Source: CAD feature listing. Evaluate the final solid. Frame: model axes, mm. A direction names the side the tool comes from. Give positions to 0.01 mm unless a question says otherwise; leave off trailing zeros. Write each loop counter-clockwise with the first axis right and the second up, starting at its lowest first coordinate (ties: lowest second). Pieces come first, ordered by that corner, then holes. Notation, with made-up numbers: (-36.75, 13) -> (22.25, 13) arc R15 cw to (22.25, 17) -> close; hole circle Ø10 at (-8, 9.25). An arc over 180 degrees is marked (long way). Answer as a JSON object with one key per item and string values. Group by question number.
Item 1: First-contact query: pin 1 Ø1.5 at (x, y) = (-183.5, 3.5) entering from -Z; pin 2 Ø1.5 at (x, y) = (132, 2) entering from +Z; pin 3 Ø3 at (x, z) = (-211.5, -104.5) entering from -Y. Flat tips, straight axial feed; report the tip coordinate or a pass-through.
Item 2: Section query A-A on x = 87.5. Return the cut outline in (y, z).
Item 3: Section query C-C on y = 4.1. Give the number of separate pieces and of enclosed holes in the cut face, plus the area to 3 significant figures.
Item 4: Ray query, probe 1 along Z at (x, y) = (-6, 3.85); probe 2 along X at (y, z) = (4.05, 16); probe 3 along X at (y, z) = (4.35, 125). Return the intervals inside material, ascending. Write a range as from..to.
Item 5: Pull-direction query (Z, two-part tool) for faces 3 (the face through (-193.081, 2.465, 118.033)), 4 (the face through (-174.6, 2.46, -43.16)), 5 (the face through (-41, 0, 72)), 6 (the face through (241.15, 2.46, -140.99)); classes: pulls with the +Z half, pulls with the -Z half, needs draft (parallel to the pull), parting line crosses it, or undercut.
Item 6: Access query for faces 1 (the face through (-41, 5, 72)), 2 (the face through (-217.63, 2.46, 81.57)). Directions: +Z, -Z, +X, -X, +Y, -Y. A direction counts if a zero-diameter tool reaches every point of the face in a straight line with its end or side. Return the directions, or none.
Item 7: Section query B-B on z = 16. Return the cut outline in (x, y), plus the area to 3 significant figures.
from build123d import *

# Parameters (mm, degrees)
ESQUISSE1_R        = 1.75
ESQUISSE1_R_2      = 11.5
ESQUISSE1_R_3      = 2.25
BOSS_EXTRU_1_DEPTH = 5


with BuildPart() as part:
    # Esquisse1 → Boss.-Extru.1 (new body)
    with BuildSketch(Plane(origin=(0, 0, 0), x_dir=(1, 0, 0), z_dir=(0, 1, 0))):
        with BuildLine():
            Line((-196.5, -144), (196.5, -144))
            ThreePointArc((196.5, -144), (201.644957554, -145.425070743), (205.323529412, -149.294117647))
            ThreePointArc((205.323529412, -149.294117647), (256.980970389, -156.980970389), (249.294117647, -105.323529412))
            ThreePointArc((249.294117647, -105.323529412), (245.425070743, -101.644957554), (244, -96.5))
            Line((244, -96.5), (244, 134))
            ThreePointArc((244, 134), (241.071067812, 141.071067812), (234, 144))
            Line((234, 144), (39.764934301, 144))
            ThreePointArc((39.764934301, 144), (34.076969712, 145.775216792), (30.408479172, 150.470588235))
            ThreePointArc((30.408479172, 150.470588235), (0, 171.5), (-30.408479172, 150.470588235))
            ThreePointArc((-30.408479172, 150.470588235), (-34.076969712, 145.775216792), (-39.764934301, 144))
            Line((-39.764934301, 144), (-234, 144))
            ThreePointArc((-234, 144), (-241.071067812, 141.071067812), (-244, 134))
            Line((-244, 134), (-244, -96.5))
            ThreePointArc((-244, -96.5), (-245.425070743, -101.644957554), (-249.294117647, -105.323529412))
            ThreePointArc((-249.294117647, -105.323529412), (-256.980970389, -156.980970389), (-205.323529412, -149.294117647))
            ThreePointArc((-205.323529412, -149.294117647), (-201.644957554, -145.425070743), (-196.5, -144))
        make_face()
        with Locations(Location((-2.5, 104.5, 0), (0, 0, 270))):  # turned: the seam where the file's is
            Circle(ESQUISSE1_R, mode=Mode.SUBTRACT)
        with Locations(Location((-211.5, 104.5, 0), (0, 0, 270))):  # turned: the seam where the file's is
            Circle(ESQUISSE1_R, mode=Mode.SUBTRACT)
        with Locations(Location((211.5, 104.5, 0), (0, 0, 90))):  # turned: the seam where the file's is
            Circle(ESQUISSE1_R, mode=Mode.SUBTRACT)
        with Locations(Location((2.5, 104.5, 0), (0, 0, 270))):  # turned: the seam where the file's is
            Circle(ESQUISSE1_R, mode=Mode.SUBTRACT)
        with Locations(Location((2.5, -104.5, 0), (0, 0, 90))):  # turned: the seam where the file's is
            Circle(ESQUISSE1_R, mode=Mode.SUBTRACT)
        with Locations(Location((-2.5, -104.5, 0), (0, 0, 90))):  # turned: the seam where the file's is
            Circle(ESQUISSE1_R, mode=Mode.SUBTRACT)
        with Locations(Location((-211.5, -104.5, 0), (0, 0, 90))):  # turned: the seam where the file's is
            Circle(ESQUISSE1_R, mode=Mode.SUBTRACT)
        with Locations(Location((211.5, -104.5, 0), (0, 0, 270))):  # turned: the seam where the file's is
            Circle(ESQUISSE1_R, mode=Mode.SUBTRACT)
        with Locations(Location((0, 139, 0), (0, 0, 270))):  # turned: the seam where the file's is
            Circle(ESQUISSE1_R_2, mode=Mode.SUBTRACT)
        with Locations(Location((-234, -134, 0), (0, 0, 270))):  # turned: the seam where the file's is
            Circle(ESQUISSE1_R_2, mode=Mode.SUBTRACT)
        with Locations(Location((234, -134, 0), (0, 0, 270))):  # turned: the seam where the file's is
            Circle(ESQUISSE1_R_2, mode=Mode.SUBTRACT)
        with Locations(Location((-11.787470042, 127.212529958, 0), (0, 0, 270))):  # turned: the seam where the file's is
            Circle(ESQUISSE1_R_3, mode=Mode.SUBTRACT)
        with Locations(Location((-11.787470042, 150.787470042, 0), (0, 0, 270))):  # turned: the seam where the file's is
            Circle(ESQUISSE1_R_3, mode=Mode.SUBTRACT)
        with Locations(Location((11.787470042, 150.787470042, 0), (0, 0, 270))):  # turned: the seam where the file's is
            Circle(ESQUISSE1_R_3, mode=Mode.SUBTRACT)
        with Locations(Location((11.787470042, 127.212529958, 0), (0, 0, 270))):  # turned: the seam where the file's is
            Circle(ESQUISSE1_R_3, mode=Mode.SUBTRACT)
        with Locations(Location((-234, -117.33, 0), (0, 0, 270))):  # turned: the seam where the file's is
            Circle(ESQUISSE1_R_3, mode=Mode.SUBTRACT)
        with Locations(Location((-217.33, -134, 0), (0, 0, 270))):  # turned: the seam where the file's is
            Circle(ESQUISSE1_R_3, mode=Mode.SUBTRACT)
        with Locations(Location((-234, -150.67, 0), (0, 0, 270))):  # turned: the seam where the file's is
            Circle(ESQUISSE1_R_3, mode=Mode.SUBTRACT)
        with Locations(Location((-250.67, -134, 0), (0, 0, 270))):  # turned: the seam where the file's is
            Circle(ESQUISSE1_R_3, mode=Mode.SUBTRACT)
        with Locations(Location((234, -117.33, 0), (0, 0, 270))):  # turned: the seam where the file's is
            Circle(ESQUISSE1_R_3, mode=Mode.SUBTRACT)
        with Locations(Location((250.67, -134, 0), (0, 0, 270))):  # turned: the seam where the file's is
            Circle(ESQUISSE1_R_3, mode=Mode.SUBTRACT)
        with Locations(Location((234, -150.67, 0), (0, 0, 270))):  # turned: the seam where the file's is
            Circle(ESQUISSE1_R_3, mode=Mode.SUBTRACT)
        with Locations(Location((217.33, -134, 0), (0, 0, 270))):  # turned: the seam where the file's is
            Circle(ESQUISSE1_R_3, mode=Mode.SUBTRACT)
        with BuildLine():
            Line((-190.881530392, 107.422917163), (-125.788799552, 32.872268168))
            ThreePointArc((-125.788799552, 32.872268168), (-118.210341928, 29.449455568), (-110.663506177, 32.94143727))
            Line((-110.663506177, 32.94143727), (-46.762949895, 107.492086265))
            ThreePointArc((-46.762949895, 107.492086265), (-45.270386934, 118.178568095), (-54.355515919, 124))
            Line((-54.355515919, 124), (-183.34880304, 124))
            ThreePointArc((-183.34880304, 124), (-192.452945734, 118.13697786), (-190.881530392, 107.422917163))
        make_face(mode=Mode.SUBTRACT)
        with BuildLine():
            Line((54.355515919, 124), (183.34880304, 124))
            ThreePointArc((183.34880304, 124), (192.452945734, 118.13697786), (190.881530392, 107.422917163))
            Line((190.881530392, 107.422917163), (125.788799552, 32.872268168))
            ThreePointArc((125.788799552, 32.872268168), (118.210341928, 29.449455568), (110.663506177, 32.94143727))
            Line((110.663506177, 32.94143727), (46.762949895, 107.492086265))
            ThreePointArc((46.762949895, 107.492086265), (45.270386934, 118.178568095), (54.355515919, 124))
        make_face(mode=Mode.SUBTRACT)
        with BuildLine():
            Line((-183.930198367, -124), (-50.65119696, -124))
            ThreePointArc((-50.65119696, -124), (-41.547054266, -118.13697786), (-43.118469608, -107.422917163))
            Line((-43.118469608, -107.422917163), (-110.373862185, -30.395373528))
            ThreePointArc((-110.373862185, -30.395373528), (-117.95231981, -26.972560928), (-125.49915556, -30.46454263))
            Line((-125.49915556, -30.46454263), (-191.52276439, -107.492086265))
            ThreePointArc((-191.52276439, -107.492086265), (-193.015327352, -118.178568095), (-183.930198367, -124))
        make_face(mode=Mode.SUBTRACT)
        with BuildLine():
            Line((-206.407433976, -78.759811829), (-143.545283572, -5.420636357))
            ThreePointArc((-143.545283572, -5.420636357), (-141.137954159, 1.13300765), (-143.605122244, 7.664360214))
            Line((-143.605122244, 7.664360214), (-206.467272648, 79.660327344))
            ThreePointArc((-206.467272648, 79.660327344), (-217.512315937, 82.446130641), (-224, 73.083244507))
            Line((-224, 73.083244507), (-224, -72.251898095))
            ThreePointArc((-224, -72.251898095), (-217.469462477, -81.630748244), (-206.407433976, -78.759811829))
        make_face(mode=Mode.SUBTRACT)
        with BuildLine():
            Line((16.237050105, 97.007913735), (92.617378166, 7.897530997))
            ThreePointArc((92.617378166, 7.897530997), (95.024707579, 1.343886989), (92.557539494, -5.187465575))
            Line((92.557539494, -5.187465575), (12.325560242, -97.077082837))
            ThreePointArc((12.325560242, -97.077082837), (8.929810751, -99.604142694), (4.792832891, -100.5))
            Line((4.792832891, -100.5), (-3.508962205, -100.5))
            ThreePointArc((-3.508962205, -100.5), (-7.610068471, -99.620357855), (-10.989673554, -97.136185479))
            Line((-10.989673554, -97.136185479), (-92.505523491, -5.246568217))
            ThreePointArc((-92.505523491, -5.246568217), (-95.024450072, 1.304521568), (-92.617378166, 7.897530997))
            Line((-92.617378166, 7.897530997), (-16.237050105, 97.007913735))
            ThreePointArc((-16.237050105, 97.007913735), (-12.823052176, 99.585128985), (-8.644484081, 100.5))
            Line((-8.644484081, 100.5), (8.644484081, 100.5))
            ThreePointArc((8.644484081, 100.5), (12.823052176, 99.585128985), (16.237050105, 97.007913735))
        make_face(mode=Mode.SUBTRACT)
        with BuildLine():
            Line((224, 73.083244507), (224, -72.251898095))
            ThreePointArc((224, -72.251898095), (217.469462477, -81.630748244), (206.407433976, -78.759811829))
            Line((206.407433976, -78.759811829), (143.545283572, -5.420636357))
            ThreePointArc((143.545283572, -5.420636357), (141.137954159, 1.13300765), (143.605122244, 7.664360214))
            Line((143.605122244, 7.664360214), (206.467272648, 79.660327344))
            ThreePointArc((206.467272648, 79.660327344), (217.512315937, 82.446130641), (224, 73.083244507))
        make_face(mode=Mode.SUBTRACT)
        with BuildLine():
            Line((125.49915556, -30.46454263), (191.52276439, -107.492086265))
            ThreePointArc((191.52276439, -107.492086265), (193.015327352, -118.178568095), (183.930198367, -124))
            Line((183.930198367, -124), (50.65119696, -124))
            ThreePointArc((50.65119696, -124), (41.547054266, -118.13697786), (43.118469608, -107.422917163))
            Line((43.118469608, -107.422917163), (110.373862185, -30.395373528))
            ThreePointArc((110.373862185, -30.395373528), (117.95231981, -26.972560928), (125.49915556, -30.46454263))
        make_face(mode=Mode.SUBTRACT)
    extrude(amount=BOSS_EXTRU_1_DEPTH)


solid = part.part
Worked answers:
{
 "1": {"pin 1": "z = -144", "pin 2": "z = 144", "pin 3": "through"},
 "2": {"outline": "(0, -144) -> (5, -144) -> (5, -124) -> (0, -124) -> close; (0, -59.97) -> (5, -59.97) -> (5, -13.87) -> (0, -13.87) -> close; (0, 10.98) -> (5, 10.98) -> (5, 56.59) -> (0, 56.59) -> close; (0, 124) -> (5, 124) -> (5, 144) -> (0, 144) -> close"},
 "3": {"separate pieces": "1", "enclosed holes": "30", "area": "71,000 mm^2"},
 "4": {"probe 1": "-170.94..-148.81, -129.19..-100.5, 100.18..144", "probe 2": "-244..-224, -152.61..-82.97, 83.12..152.61, 224..244", "probe 3": "-265.23..-241.16, -226.84..226.84, 241.16..265.23"},
 "5": {"face 3": "undercut", "face 4": "undercut", "face 5": "needs draft", "face 6": "pulls with the -Z half"},
 "6": {"face 1": "+Z, -Z, +X, -X, +Y", "face 2": "+Y, -Y"},
 "7": {"outline": "(-244, 0) -> (-224, 0) -> (-224, 5) -> (-244, 5) -> close; (-152.61, 0) -> (-82.97, 0) -> (-82.97, 5) -> (-152.61, 5) -> close; (83.12, 0) -> (152.61, 0) -> (152.61, 5) -> (83.12, 5) -> close; (224, 0) -> (244, 0) -> (244, 5) -> (224, 5) -> close", "area": "896 mm^2"}
}
